```python
from build123d import *

# Parameters (mm, degrees)
F1_DEPTH = 19.9644
F2_R     = 0.79375


with BuildPart() as f1:
    # F0 (on Top) → F1 (new body)
    with BuildSketch(Plane.XY):
        with BuildLine():
            Line((21.6, 0), (15.113, 0))
            ThreePointArc((15.113, 0), (0, -15.113), (-15.113, 0))
            Line((-15.113, 0), (-21.6, 0))
            ThreePointArc((-21.6, 0), (-15.2735064736, -15.2735064736), (0, -21.6))
            ThreePointArc((0, -21.6), (15.2735064736, -15.2735064736), (21.6, 0))
        make_face()
        with BuildLine():
            ThreePointArc((-15.113, 0), (0, 15.113), (15.113, 0))
            Line((15.113, 0), (21.6, 0))
            ThreePointArc((21.6, 0), (0, 21.6), (-21.6, 0))
            Line((-21.6, 0), (-15.113, 0))
        make_face()
        with BuildLine():
            Line((21.6, -21.6), (21.6, 0))
            ThreePointArc((21.6, 0), (15.2735064736, -15.2735064736), (0, -21.6))
            Line((0, -21.6), (21.6, -21.6))
        make_face()
        with BuildLine():
            ThreePointArc((0, -21.6), (-15.2735064736, -15.2735064736), (-21.6, 0))
            Line((-21.6, 0), (-21.6, -21.6))
            Line((-21.6, -21.6), (0, -21.6))
        make_face()
    extrude(amount=F1_DEPTH)

    # F2
    f2_edges = [f1.edges().sort_by_distance(p)[0] for p in [
        (0, 21.6, 0),
        (0, 21.6, 19.9644),
    ]]
    fillet(f2_edges, radius=F2_R)


solid = f1.part
```
Input: part model. Units: mm. Frame: model coordinates. Coordinates: 2 decimals unless noted, no trailing zeros. Write each loop counter-clockwise with the first axis right and the second up, starting at its lowest first coordinate (ties: lowest second). Pieces come first, ordered by that corner, then holes. Notation, with made-up numbers: (65, 75) -> (122, 75) arc R6 ccw to (122, 79) -> close; hole circle Ø6 at (41.25, 9.5). An arc over 180 degrees is marked (long way). Answer as a JSON object with one key per item and string values.
1. Section C-C on y = -1. Return the cut outline in (x, z).
Result set:
{"outline": "(-21.6, 0.79) arc R0.79 ccw to (-20.81, 0) -> (-15.08, 0) -> (-15.08, 19.96) -> (-20.81, 19.96) arc R0.79 ccw to (-21.6, 19.17) -> close; (15.08, 0) -> (20.81, 0) arc R0.79 ccw to (21.6, 0.79) -> (21.6, 19.17) arc R0.79 ccw to (20.81, 19.96) -> (15.08, 19.96) -> close"}
2. Material intervals for line 1 (Y direction, x = 0, z = 5.5); line 2 (Y direction, x = -3, z = 14.75); line 3 (X direction, y = -11.5, z = 1), sorted ascending. Write a range as from..to.
Result set:
{"line 1": "y = -21.6..-15.11, 15.11..21.6", "line 2": "y = -21.6..-14.81, 14.81..21.39", "line 3": "x = -21.6..-9.81, 9.81..21.6"}
3. First-contact query: P1, Ø5, axis at x = -4.5, z = 6, coming from the +Y side; P2, Ø8, axis at x = 13, z = 16, coming from the +Y side; P3, Ø3, axis at x = -0.5, z = 11, coming from the +Y side. Flat tips, straight axial feed; report the tip coordinate or a pass-through.
Result set:
{"P1": "stops at y = 21.51", "P2": "stops at y = 19.64", "P3": "stops at y = 21.6"}
4. Section A-A on x = 0. Return the cut outline in (y, z).
Result set:
{"outline": "(-21.6, 0) -> (-15.11, 0) -> (-15.11, 19.96) -> (-21.6, 19.96) -> close; (15.11, 0) -> (20.81, 0) arc R0.79 ccw to (21.6, 0.79) -> (21.6, 19.17) arc R0.79 ccw to (20.81, 19.96) -> (15.11, 19.96) -> close"}
5. Section B-B on z = 14.25. Return the cut outline in (x, y).
Result set:
{"outline": "(-21.6, -21.6) -> (21.6, -21.6) -> (21.6, 0) arc R21.6 ccw to (-21.6, 0) -> close; hole circle Ø30.23 at (0, 0)"}
6. Mould query, pull axis Y, two halves, no side actions, for faces 1 (the face through (9, -14, 0)), 2 (the face through (0.475, 21.595, 9.854)), 3 (the face through (11.14, 10.21, 9.84)). Classes: released by +Y, released by -Y, zero draft, split by the parting line, or undercut.
Result set:
{"face 1": "zero draft", "face 2": "released by +Y", "face 3": "undercut"}
